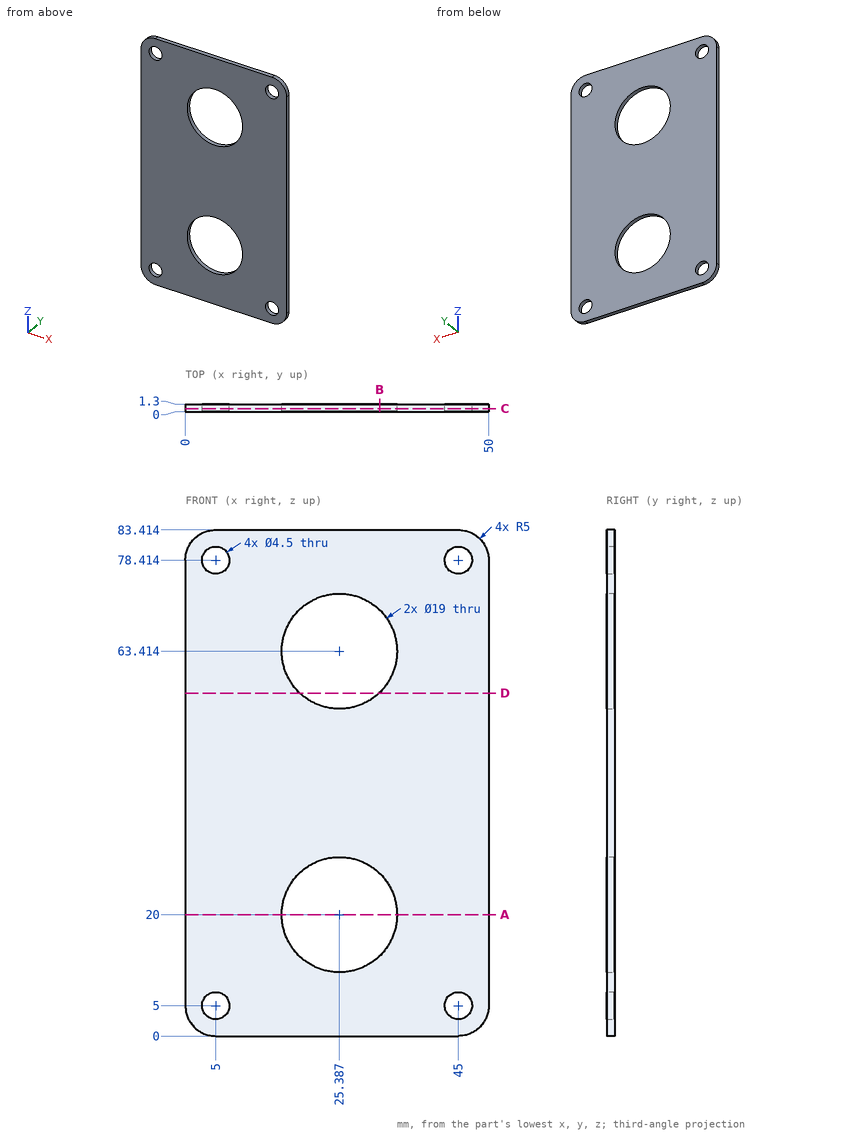
Drawing for the job (mm, zero at the part's lowest x, y, z). Round coordinates to 2 decimals unless told otherwise and drop trailing zeros. Order: outer loops, then holes, each group sorted by start corner. A loop starts at its lowest first (then second) coordinate and runs counter-clockwise, first axis right, second up. Notation, with made-up numbers: (79, 47.25) -> (116, 47.25) arc R23 ccw to (116, 56.25) -> close; hole circle Ø11 at (89, 48). An arc over 180 degrees is marked (long way). Put each result on its own line as item: value.
Q1. Pin check, flat tip, straight feed: pin 1 Ø22 at (x, z) = (25.39, 20) entering from +Y. Stop position of the tip, or through.
From the geometry:
pin 1: stops at y = 1.3
Q2. Wall check: line 1 (Z direction, x = 26, y = 1.2) (1 decimal); line 2 (X direction, y = 0.4, z = 5); line 3 (Z direction, x = 6, y = 0.25) (1 decimal). Give the ranges that are in metal, low to high. Write a range as [from, to].
From the geometry:
line 1: z = [0, 10.5], [29.5, 53.9], [72.9, 83.4]
line 2: x = [0, 2.75], [7.25, 42.75], [47.25, 50]
line 3: z = [0, 3], [7, 76.4], [80.4, 83.4]
Q3. Band-saw the part on C-C (y = 0.55). Give the cut face in (x, z), and give its area (3 significant figures).
From the geometry:
outline: (0, 5) arc R5 ccw to (5, 0) -> (45, 0) arc R5 ccw to (50, 5) -> (50, 78.41) arc R5 ccw to (45, 83.41) -> (5, 83.41) arc R5 ccw to (0, 78.41) -> close; hole circle Ø4.5 at (5, 5); hole circle Ø4.5 at (5, 78.41); hole circle Ø19 at (25.39, 20); hole circle Ø19 at (25.39, 63.41); hole circle Ø4.5 at (45, 5); hole circle Ø4.5 at (45, 78.41)
area: 3,520 mm2
Q4. Band-saw the part on A-A (z = 20). Give the cut face in (x, y), and give its area (3 significant figures).
From the geometry:
outline: (0, 0) -> (15.89, 0) -> (15.89, 1.3) -> (0, 1.3) -> close; (34.89, 0) -> (50, 0) -> (50, 1.3) -> (34.89, 1.3) -> close
area: 40.3 mm2
Q5. Band-saw the part on D-D (z = 56.5). Give the cut face in (x, y).
From the geometry:
outline: (0, 0) -> (18.87, 0) -> (18.87, 1.3) -> (0, 1.3) -> close; (31.9, 0) -> (50, 0) -> (50, 1.3) -> (31.9, 1.3) -> close
Q6. Band-saw the part on B-B (x = 32). Give the cut face in (y, z) (1 decimal).
From the geometry:
outline: (0, 0) -> (1.3, 0) -> (1.3, 13.2) -> (0, 13.2) -> close; (0, 26.8) -> (1.3, 26.8) -> (1.3, 56.6) -> (0, 56.6) -> close; (0, 70.2) -> (1.3, 70.2) -> (1.3, 83.4) -> (0, 83.4) -> close
